Verification items for the finished model (mm, model axes). A direction names the side the tool comes from. Round coordinates to 2 decimals unless told otherwise and drop trailing zeros. Order: outer loops, then holes, each group sorted by start corner. A loop starts at its lowest first (then second) coordinate and runs counter-clockwise, first axis right, second up. Notation, with made-up numbers: M 32.5,10 L 83.5,10 A10 ccw 83.5,21 Z; hole C -21.75,28 d10. An arc over 180 degrees is marked long. One line per item, written item: value. Start each with the question number.
from build123d import *

# Parameters (mm, degrees)
F0_R     = 1.25
F0_R_2   = 5.5
F1_DEPTH = 3
F2_W     = 3.325
F2_H     = 2.6
F3_DEPTH = 16.4
F4_SIZE  = 2
F5_R     = 5


with BuildPart() as f1:
    # F0 (on Top) → F1 (new body)
    with BuildSketch(Plane.XY):
        with BuildLine():
            Line((17.074093, -19.419351), (17.074093, 9.280649))
            Line((17.074093, 9.280649), (13.749093, 9.280649))
            Line((13.749093, 9.280649), (13.749093, -4.019351))
            Line((13.749093, -4.019351), (3.249093, -4.019351))
            Line((3.249093, -4.019351), (3.249093, -5.947351))
            ThreePointArc((3.249093, -5.947351), (-0.850907, -10.047351), (-4.950907, -5.947351))
            Line((-4.950907, -5.947351), (-4.950907, -4.019351))
            Line((-4.950907, -4.019351), (-30.900907, -4.019351))
            Line((-30.900907, -4.019351), (-30.900907, -5.947351))
            ThreePointArc((-30.900907, -5.947351), (-35.000907, -10.047351), (-39.100907, -5.947351))
            Line((-39.100907, -5.947351), (-39.100907, -4.019351))
            Line((-39.100907, -4.019351), (-49.600907, -4.019351))
            Line((-49.600907, -4.019351), (-49.600907, 25.180649))
            Line((-49.600907, 25.180649), (-39.100907, 25.180649))
            Line((-39.100907, 25.180649), (-39.100907, 27.108649))
            ThreePointArc((-39.100907, 27.108649), (-35.000907, 31.208649), (-30.900907, 27.108649))
            Line((-30.900907, 27.108649), (-30.900907, 25.180649))
            Line((-30.900907, 25.180649), (-4.950907, 25.180649))
            Line((-4.950907, 25.180649), (-4.950907, 27.108649))
            ThreePointArc((-4.950907, 27.108649), (-0.850907, 31.208649), (3.249093, 27.108649))
            Line((3.249093, 27.108649), (3.249093, 25.180649))
            Line((3.249093, 25.180649), (13.749093, 25.180649))
            Line((13.749093, 25.180649), (13.749093, 11.880649))
            Line((13.749093, 11.880649), (17.074093, 11.880649))
            Line((17.074093, 11.880649), (17.074093, 40.580649))
            Line((17.074093, 40.580649), (-52.925907, 40.580649))
            Line((-52.925907, 40.580649), (-52.925907, -19.419351))
            Line((-52.925907, -19.419351), (17.074093, -19.419351))
        make_face()
        with Locations((-44.350907, -11.719351)):
            Circle(F0_R, mode=Mode.SUBTRACT)
        with Locations((8.499093, -11.719351)):
            Circle(F0_R, mode=Mode.SUBTRACT)
        with Locations((-44.350907, 32.880649)):
            Circle(F0_R, mode=Mode.SUBTRACT)
        with Locations((8.499093, 32.880649)):
            Circle(F0_R, mode=Mode.SUBTRACT)
        with BuildLine():
            Line((13.749093, -4.019351), (13.749093, 9.280649))
            Line((13.749093, 9.280649), (13.749093, 11.880649))
            Line((13.749093, 11.880649), (13.749093, 25.180649))
            Line((13.749093, 25.180649), (3.249093, 25.180649))
            Line((3.249093, 25.180649), (3.249093, 27.108649))
            ThreePointArc((3.249093, 27.108649), (-0.850907, 31.208649), (-4.950907, 27.108649))
            Line((-4.950907, 27.108649), (-4.950907, 25.180649))
            Line((-4.950907, 25.180649), (-30.900907, 25.180649))
            Line((-30.900907, 25.180649), (-30.900907, 27.108649))
            ThreePointArc((-30.900907, 27.108649), (-35.000907, 31.208649), (-39.100907, 27.108649))
            Line((-39.100907, 27.108649), (-39.100907, 25.180649))
            Line((-39.100907, 25.180649), (-49.600907, 25.180649))
            Line((-49.600907, 25.180649), (-49.600907, -4.019351))
            Line((-49.600907, -4.019351), (-39.100907, -4.019351))
            Line((-39.100907, -4.019351), (-39.100907, -5.947351))
            ThreePointArc((-39.100907, -5.947351), (-35.000907, -10.047351), (-30.900907, -5.947351))
            Line((-30.900907, -5.947351), (-30.900907, -4.019351))
            Line((-30.900907, -4.019351), (-4.950907, -4.019351))
            Line((-4.950907, -4.019351), (-4.950907, -5.947351))
            ThreePointArc((-4.950907, -5.947351), (-0.850907, -10.047351), (3.249093, -5.947351))
            Line((3.249093, -5.947351), (3.249093, -4.019351))
            Line((3.249093, -4.019351), (13.749093, -4.019351))
        make_face()
        with Locations((2.749093, 10.580649)):
            Circle(F0_R_2, mode=Mode.SUBTRACT)
    extrude(amount=F1_DEPTH)

    # F2 (on face) → F3 (join)
    with BuildSketch(Plane(origin=(0, 0, 0), x_dir=(1, 0, 0), z_dir=(0, 0, -1))):
        with Locations((15.411593, -10.580649)):
            Rectangle(F2_W, F2_H)
    extrude(amount=-F3_DEPTH)

    # F4
    f4_edges = [f1.edges().sort_by_distance(p)[0] for p in [
        (-45.600907, -11.719351, 0),
        (-45.600907, 32.880649, 0),
        (7.249093, 32.880649, 0),
        (7.249093, -11.719351, 0),
    ]]
    chamfer(f4_edges, length=F4_SIZE)

    # F5
    f5_edges = [f1.edges().sort_by_distance(p)[0] for p in [
        (-52.925907, -19.419351, 1.5),
        (17.074093, -19.419351, 1.5),
        (17.074093, 40.580649, 1.5),
        (-52.925907, 40.580649, 1.5),
    ]]
    fillet(f5_edges, radius=F5_R)


solid = f1.part
1. Section check A-A (y = 14.5). Record the cut outline in (x, z), and give its area (3 significant figures).
2. Section check B-B (x = 0.5). Record the cut outline in (y, z), and give its area (3 significant figures).
3. Section check D-D (y = 26.5). Record the cut outline in (x, z), and give its area (3 significant figures).
4. Section check C-C (z = 11). Record the cut outline in (x, y), and give its area (4 significant figures).
5. Scan lines: line 1 along Z through (x, y) = (-27, -4.5); line 2 along X through (y, z) = (6, 2); line 3 along X through (y, z) = (12.5, 2.5). Record each from-to range of solid material in increasing order.
6. Tool access check on faces 4 (the face through (13.749, 11, 10)), 5 (the face through (17.074, 10, 3)), 6 (the face through (15, 9.281, 10)). Record the directions out of +Z, -Z, +X, -X, +Y, -Y that give a thin tool (end or side, any length) a straight path to the whole face; none if there is none.
7. Draft check along X on faces 1 (the face through (15, 11.881, 10)), 2 (the face through (-51.5, -17.916, 1.521)), 3 (the face through (9.171, -10.665, 2.493)). Enter one of: released by +X, released by -X, zero draft, split by the parting line, or undercut.
8. Depth check by flat-ended pin: pin 1 (2.5 mm diameter, centred on x = 15, z = 13, fed in from -Y); pin 2 (9 mm diameter, centred on x = 2.75, y = 10.58, fed in from +Z); pin 3 (3 mm diameter, centred on x = 8.5, y = -11.72, fed in from -Z); pin 4 (2 mm diameter, centred on x = -4.5, y = 12.5, fed in from +Z). Enter the tip coordinate at first touch or a pass-through.
Geometry check:
1. outline: M -52.93,0 L -1.11,0 L -1.11,3 L -52.93,3 Z; M 6.61,0 L 17.07,0 L 17.07,3 L 6.61,3 Z
1. area: 187 mm²
2. outline: M -19.42,0 L 5.56,0 L 5.56,3 L -19.42,3 Z; M 15.6,0 L 40.58,0 L 40.58,3 L 15.6,3 Z
2. area: 150 mm²
3. outline: M -52.93,0 L 17.07,0 L 17.07,3 L -52.93,3 Z
3. area: 210 mm²
4. outline: M 13.75,9.28 L 17.07,9.28 L 17.07,11.88 L 13.75,11.88 Z
4. area: 8.645 mm²
5. line 1: z = 0 to 3
5. line 2: x = -52.93 to -0.3, 5.79 to 17.07
5. line 3: x = -52.93 to -2.41, 7.9 to 17.07
6. face 4: +Z, -X, +Y, -Y
6. face 5: +Z, -Z, +X, +Y, -Y
6. face 6: +Z, +X, -X, -Y
7. face 1: zero draft
7. face 2: released by -X
7. face 3: undercut
8. pin 1: stops at y = 9.28
8. pin 2: passes through
8. pin 3: stops at z = 1.75
8. pin 4: stops at z = 3
